Input: dimensioned drawing with shaded views. Units: mm. Origin: part minimum x, y, z. A direction names the side the tool comes from. Round coordinates to 2 decimals unless told otherwise and drop trailing zeros. Write each loop counter-clockwise with the first axis right and the second up, starting at its lowest first coordinate (ties: lowest second). Pieces come first, ordered by that corner, then holes. Notation, with made-up numbers: (-25.75, 7) - (3.25, 7) arc R16 ccw to (3.25, 18) - close; hole circle Ø8 at (61, 71). An arc over 180 degrees is marked (long way). Use one line per item in the form item = value.
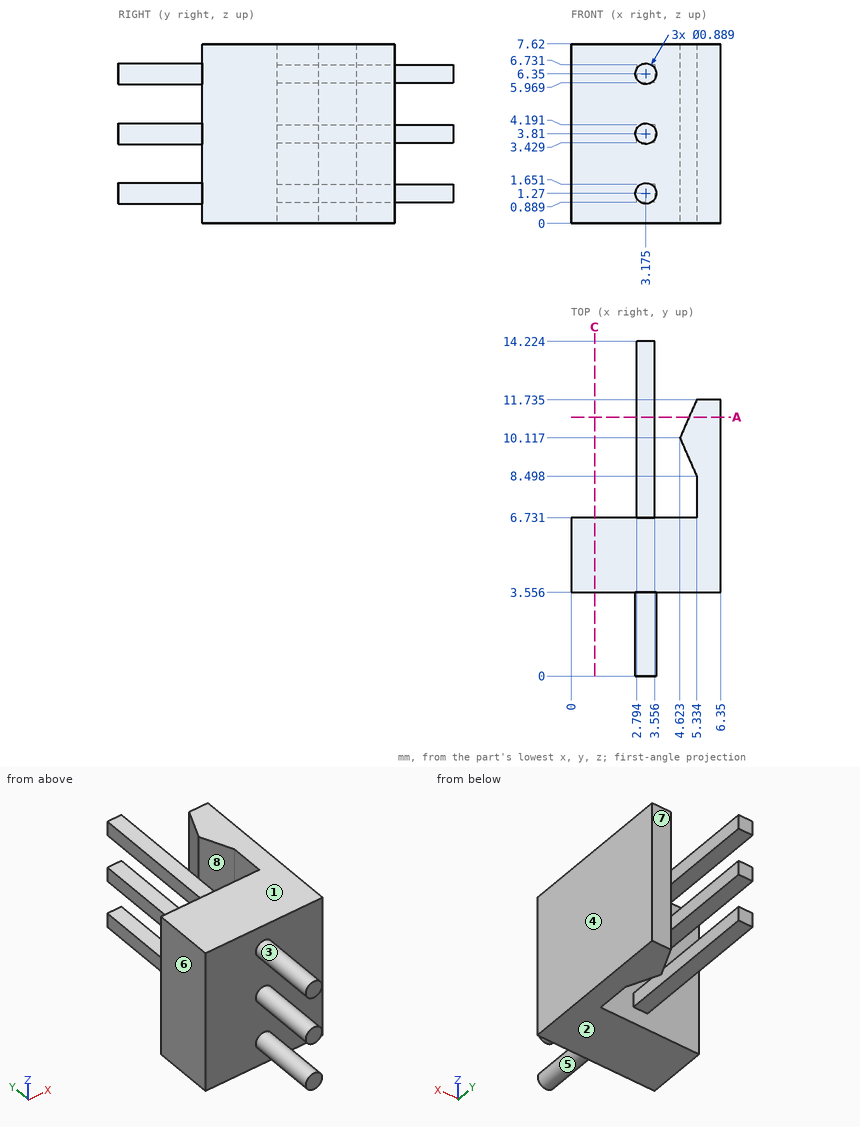
(1) Access query for the marked faces 4, 5, 6, 7 and 8. Directions: +Z, -Z, +X, -X, +Y, -Y. A direction counts if a zero-diameter tool reaches every point of the face in a straight line with its end or side. Return the directions, or none.
Derived:
face_4 = +Z, -Z, +X, +Y, -Y
face_5 = -Y
face_6 = +Z, -Z, -X, +Y, -Y
face_7 = +Z, -Z, +X, +Y
face_8 = +Z, -Z
(2) Cut plane C-C on x = 1. Output: boundary loops of the cut face in (y, z) (1 decimal).
Derived:
outline = (3.6, 0) - (6.7, 0) - (6.7, 7.6) - (3.6, 7.6) - close
(3) Cut plane A-A on y = 11. Count the separate pieces of the cut face and the enclosed holes in it.
Derived:
separate_pieces = 4
enclosed_holes = 0
(4) Draft query along Z for the marked faces 1, 2 and 3. Return one class per face: released by +Z, released by -Z, zero draft, split by the parting line, or undercut.
Derived:
face_1 = released by +Z
face_2 = released by -Z
face_3 = undercut
(5) Material intervals for L1, parallel to Y at x = 4.5, z = 6.75 (1 decimal); L2, parallel to X at y = 12, z = 6.5 (1 decimal); L3, parallel to Y at x = 6, z = 4.75 (1 decimal), sorted ascending.
Derived:
L1 = 3.6 to 6.7
L2 = 2.8 to 3.6
L3 = 3.6 to 11.7
(6) First-contact query: pin 1 Ø1 at (x, z) = (5.5, 6.5) entering from +Y (1 decimal); pin 2 Ø0.8 at (x, y) = (3, 12) entering from -Z; pin 3 Ø0.8 at (y, z) = (9.5, 1) entering from -X. Flat tips, straight axial feed; report the tip coordinate or a pass-through.
Derived:
pin_1 = 11.7
pin_2 = 0.89
pin_3 = 2.79
